Source: CAD feature listing. Evaluate the final solid. Frame: model axes, mm. Face numbers are marked on the shaded views. Round coordinates to 2 decimals unless told otherwise and drop trailing zeros. Order: outer loops, then holes, each group sorted by start corner. A loop starts at its lowest first (then second) coordinate and runs counter-clockwise, first axis right, second up. Notation, with made-up numbers: (-36.5, 23.25) -> (6.5, 23.25) arc R16 cw to (6.5, 44.25) -> close; hole circle Ø6 at (10, 12). An arc over 180 degrees is marked (long way). Use a Markdown table: item, result. Add a question column.
```python
from build123d import *

# Parameters (mm, degrees)
F1_DEPTH  = 20
F3_W      = 22.4105001092
F3_H      = 37
F3_W_2    = 48.6809194684
F4_DEPTH  = 28
F5_R      = 2
F6_DEPTH  = 2
F7_DEPTH  = 40
F8_DEPTH  = 2
F10_DEPTH = 2
F11_R     = 13.5
F12_DEPTH = 5


with BuildPart() as f1:
    # F0 (on Front) → F1 (new body)
    with BuildSketch(Plane.XZ):
        Polygon((-23.9105001092, 33.5152801126), (-23.9105001092, 0), (50.0319972634, 0), (50.1809194684, 17.9111845791), (0, 33.5152801126), align=None)
    extrude(amount=F1_DEPTH)

    # F2: F1 across face


with BuildPart() as f1_1:
    add(f1.part)
    add(f1.part.mirror(Plane(origin=(9.3059845029, 0, 14.6000769053), x_dir=(1, 0, 0), z_dir=(0, 1, 0))))

    # F3 (on face) → F4 (cut)
    with BuildSketch(Plane.XY.offset(33.5152801126)):
        with Locations((-11.2052500546, 0)):
            Rectangle(F3_W, F3_H)
        with Locations((24.3404597342, 0)):
            Rectangle(F3_W_2, F3_H)
    extrude(amount=-F4_DEPTH, mode=Mode.SUBTRACT)

    # F5 (on face) → F6 (join)
    with BuildSketch(Plane.XZ.offset(20)):
        Polygon((14.9534574564, 13.3521119993), (14.4816109652, 16.0829288897), (11.8807309195, 17.0397062869), (9.7516973649, 15.2656667936), (10.2235438561, 12.5348499033), (12.8244239018, 11.5780725061), align=None)
        with Locations((12.3525774106, 14.3088893965)):
            Circle(F5_R, mode=Mode.SUBTRACT)
    extrude(amount=F6_DEPTH)

    # F7 (add): a face of the model
    f7_faces = [f1_1.faces().sort_by_distance(p)[0] for p in [
        (12.3525774106, -20, 14.3088893965),
    ]]
    extrude(f7_faces, amount=-F7_DEPTH)

    # F8 (add): a face of the model
    f8_faces = [f1_1.faces().sort_by_distance(p)[0] for p in [
        (12.3525774106, -20, 14.3088893965),
    ]]
    extrude(f8_faces, amount=F8_DEPTH)

    # F9 (on face) → F10 (join)
    with BuildSketch(Plane(origin=(0, 20, 0), x_dir=(-1, 0, 0), z_dir=(0, 1, 0))):
        Polygon((-8.9518631259, 11.5546170938), (-8.7388157611, 14.7756681167), (-11.4218040914, 16.5706980583), (-14.3178397865, 15.144676977), (-14.5308871513, 11.9236259541), (-11.847898821, 10.1285960125), align=None)
    extrude(amount=F10_DEPTH)

    # F11 (on face) → F12 (cut)
    with BuildSketch(Plane(origin=(-23.9105001092, 0, 0), x_dir=(0, -1, 0), z_dir=(-1, 0, 0))):
        with Locations((0, 17.928481102)):
            Circle(F11_R)
    extrude(amount=-F12_DEPTH, mode=Mode.SUBTRACT)


solid = f1_1.part
```
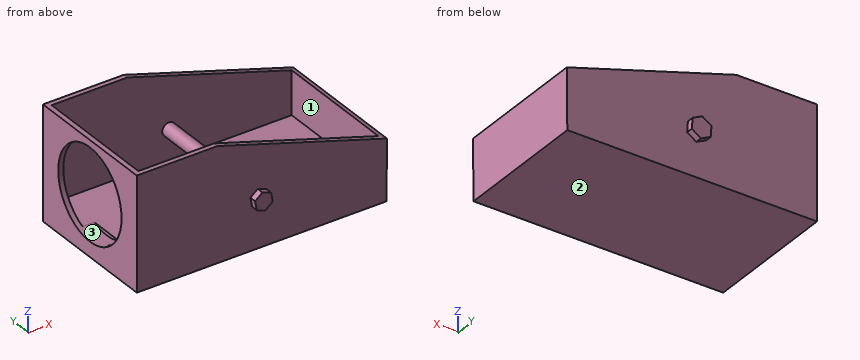
1) Section D-D on y = 0. Output: boundary loops of the cut face in (x, z).
2) Line query: probe 1 along Y at (x, z) = (-2.5, 15.5); probe 2 along Z at (x, y) = (-22.8, 0); probe 3 along Z at (x, y) = (45.5, 12.5). Output: solid intervals per line, ascending. Write a range as from..to.
3) Section B-B on x = -10. Output: boundary loops of the cut face in (y, z), then the cut area to 3 significant figures.
4) Draft query along Z for the marked faces 1, 2 and 3. Return one class per face: pulls with the +Z half, pulls with the -Z half, needs draft (parallel to the pull), parting line crosses it, or undercut.
5) Section A-A on y = -10. Output: boundary loops of the cut face in (x, z).
6) First-contact query: pin 1 Ø14 at (x, z) = (29, 19.5) entering from +Y; pin 2 Ø6.5 at (y, z) = (-5, 12) entering from -X; pin 3 Ø6 at (x, y) = (26, 4) entering from -Z; pin 4 Ø11 at (x, y) = (-2.5, -1.5) entering from +Z. Flat tips, straight axial feed; report the tip coordinate or a pass-through.
7) Section C-C on z = 25.5. Output: boundary loops of the cut face in (x, y), then the cut area to 3 significant figures.
Conclusion:
| question | item | result |
|---|---|---|
| 1 | outline | (-23.91, 0) -> (50.03, 0) -> (50.18, 17.91) -> (48.68, 18.38) -> (48.68, 5.52) -> (-18.91, 5.52) -> (-18.91, 4.43) -> (-23.91, 4.43) -> close; (-23.91, 31.43) -> (-22.41, 31.43) -> (-22.41, 33.52) -> (-23.91, 33.52) -> close; circle Ø4 at (12.35, 14.31) |
| 2 | probe 1 | y = -20..-18.5, 18.5..20 |
| 2 | probe 2 | z = 0..4.43, 31.43..33.52 |
| 2 | probe 3 | z = 0..5.52 |
| 3 | outline | (-20, 0) -> (20, 0) -> (20, 33.52) -> (18.5, 33.52) -> (18.5, 5.52) -> (-18.5, 5.52) -> (-18.5, 33.52) -> (-20, 33.52) -> close |
| 3 | area | 305 mm^2 |
| 4 | face 1 | needs draft |
| 4 | face 2 | pulls with the -Z half |
| 4 | face 3 | undercut |
| 5 | outline | (-23.91, 0) -> (50.03, 0) -> (50.18, 17.91) -> (48.68, 18.38) -> (48.68, 5.52) -> (-22.41, 5.52) -> (-22.41, 8.86) -> (-23.91, 8.86) -> close; (-23.91, 27) -> (-22.41, 27) -> (-22.41, 33.52) -> (-23.91, 33.52) -> close; circle Ø4 at (12.35, 14.31) |
| 6 | pin 1 | stops at y = 20 |
| 6 | pin 2 | stops at x = 10.35 |
| 6 | pin 3 | stops at z = 0 |
| 6 | pin 4 | stops at z = 5.52 |
| 7 | outline | (-23.91, -20) -> (25.78, -20) -> (25.78, -18.5) -> (-22.41, -18.5) -> (-22.41, -11.18) -> (-23.91, -11.18) -> close; (-23.91, 11.18) -> (-22.41, 11.18) -> (-22.41, 18.5) -> (25.78, 18.5) -> (25.78, 20) -> (-23.91, 20) -> close |
| 7 | area | 171 mm^2 |
